Work out the finished part from the listing and answer in its coordinate system (mm). A direction names the side the tool comes from. Coordinates: 2 decimals unless noted, no trailing zeros. Write each loop counter-clockwise with the first axis right and the second up, starting at its lowest first coordinate (ties: lowest second). Pieces come first, ordered by that corner, then holes. Notation, with made-up numbers: (-1.75, 64.25) - (45.25, 64.25) arc R18 cw to (45.25, 76.25) - close; hole circle Ø4 at (43.25, 68). An arc over 180 degrees is marked (long way). Use a Markdown table: item, result. Add a question column.
(1) Given pin 1 Ø8 at (x, y) = (2.5, -25.5) entering from -Z; pin 2 Ø17 at (x, y) = (0, 0) entering from -Z; pin 3 Ø1.5 at (x, z) = (10, 2.5) entering from +Y, each flat-ended and moving along its own axis, determine where each tip first touches the part or whether it passes through.
(2) The part is cut by section D-D, the plane x = 4. Give the vertices of the cut face in (y, z) (3 decimals), then the cut area to 3 significant figures.
(3) The part is cut by section A-A, the plane z = 1.9. State how many separate pieces and enclosed holes the cut face has, then the cut area to 3 significant figures.
(4) For a pull along Y with two mould halves and no side action, classify faces 4 (the face through (-7, -35, 3.175)), 5 (the face through (0.475, -125.824, 1.61)), 6 (the face through (20.994, -97.916, 1.61)) as released by +Y, released by -Y, zero draft, split by the parting line, or undercut.
(5) A tool of negligible diameter and unlimited length cuts with its end or side. For faces 1 (the face through (-21.59, -32, 2)), 2 (the face through (-20.58, -39.69, 1.61)), 3 (the face through (-27.303, -3.698, 1.565)), from which of +Z, -Z, +X, -X, +Y, -Y can it reach the whole face along a straight path? Write none if from no direction.
(6) Find the intervals of material crossed by line 1 (Y direction, x = -10.5, z = 2.9); line 2 (Y direction, x = -9.5, z = 2.6); line 3 (Y direction, x = -16, z = 2.25), in increasing order. Write a range as from..to.
(7) The part is cut by section B-B, the plane y = -80.01. Give the vertices of the cut face in (x, z) (3 decimals).
(8) The part is cut by section C-C, the plane x = 17. Give the vertices of the cut face in (y, z) (3 decimals), then the cut area to 3 significant figures.
from build123d import *

# Parameters (mm, degrees)
SKETCH1_R            = 14.2875
SKETCH1_R_2          = 2.54
BOSS_EXTRUDE1_DEPTH  = 3.175
CUT_EXTRUDE1_DEPTH   = 162.674043733
FILLET3_R            = 6.35
BOSS_EXTRUDE3_START  = -3.175
SKETCH3_R            = 2.54
BOSS_EXTRUDE3_DEPTH  = 3.175
SKETCH6_R            = 2.54
BOSS_EXTRUDE4_DEPTH  = 3.175
FILLET2_R            = 6.35
CUT_EXTRUDE2_DEPTH   = 168.423732074
CUT_EXTRUDE3_DEPTH   = 168.423732074
CUT_EXTRUDE4_DEPTH   = 168.265702461
BOSS_EXTRUDE8_START  = -3.175
SKETCH15_R           = 2.54
BOSS_EXTRUDE8_DEPTH  = 3.175
FILLET4_R            = 2.54
BOSS_EXTRUDE9_DEPTH  = 3.175
SKETCH17_R           = 14.2875
BOSS_EXTRUDE10_DEPTH = 3.175
CUT_EXTRUDE5_DEPTH   = 131.456264953
SKETCH20_R           = 14.2875
CUT_EXTRUDE6_DEPTH   = 131.456264953
SKETCH21_R           = 2.54
CUT_EXTRUDE7_DEPTH   = 131.456264953


with BuildPart() as part:
    # Sketch1 → Boss-Extrude1 (new body)
    with BuildSketch(Plane.XY):
        with BuildLine():
            Line((-8.89, 25.4), (8.89, 25.4))
            ThreePointArc((8.89, 25.4), (17.870256121, 21.680256121), (21.59, 12.7))
            Line((21.59, 12.7), (21.59, -117.775079775))
            ThreePointArc((21.59, -117.775079775), (21.127743647, -120.388718212), (19.797058824, -122.685251408))
            Line((19.797058824, -122.685251408), (-7.952696208, -155.616779465))
            ThreePointArc((-7.952696208, -155.616779465), (-12.268297602, -157.851943494), (-16.900388255, -156.380852124))
            Line((-16.900388255, -156.380852124), (-32.439211784, -143.287061102))
            ThreePointArc((-32.439211784, -143.287061102), (-34.674375812, -138.971459708), (-33.203284443, -134.339369055))
            Line((-33.203284443, -134.339369055), (-23.382941176, -122.685251408))
            ThreePointArc((-23.382941176, -122.685251408), (-22.052256353, -120.388718212), (-21.59, -117.775079775))
            Line((-21.59, -117.775079775), (-21.59, 12.7))
            ThreePointArc((-21.59, 12.7), (-17.870256121, 21.680256121), (-8.89, 25.4))
        make_face()
        Circle(SKETCH1_R, mode=Mode.SUBTRACT)
        with Locations((0, -101.6)):
            Circle(SKETCH1_R, mode=Mode.SUBTRACT)
        with Locations((-18.532085478, -142.550133084)):
            Circle(SKETCH1_R_2, mode=Mode.SUBTRACT)
        with Locations((0, -50.8)):
            Circle(SKETCH1_R_2, mode=Mode.SUBTRACT)
    extrude(amount=BOSS_EXTRUDE1_DEPTH)

    # Sketch2 → Cut-Extrude1 (cut, through all)
    with BuildSketch(Plane.XY):
        with BuildLine():
            ThreePointArc((19.159083004, -91.647229609), (9.182340769, -50.8), (19.159083004, -9.952770391))
            ThreePointArc((19.159083004, -9.952770391), (20.973467787, -5.122670102), (21.59, 0))
            Line((21.59, 0), (27.94, 0))
            Line((27.94, 0), (27.94, -121.656687185))
            Line((27.94, -121.656687185), (-7.789552878, -164.05809836))
            Line((-7.789552878, -164.05809836), (-17.501317584, -155.874478972))
            Line((-17.501317584, -155.874478972), (16.51, -115.512152961))
            ThreePointArc((16.51, -115.512152961), (20.280273667, -109.005308906), (21.59, -101.6))
            ThreePointArc((21.59, -101.6), (20.973467787, -96.477329898), (19.159083004, -91.647229609))
        make_face()
        with BuildLine():
            Line((-21.59, -41.275), (-21.59, -60.325))
            ThreePointArc((-21.59, -60.325), (-12.065, -50.8), (-21.59, -41.275))
        make_face()
    extrude(amount=CUT_EXTRUDE1_DEPTH, mode=Mode.SUBTRACT)

    # Fillet3
    fillet3_edges = [part.edges().sort_by_distance(p)[0] for p in [
        (-21.59, -41.275, 1.5875),
        (-21.59, -60.325, 1.5875),
    ]]
    fillet(fillet3_edges, radius=FILLET3_R)

    # Sketch3 → Boss-Extrude3 (add)
    with BuildSketch(Plane.XY.offset(3.175).offset(BOSS_EXTRUDE3_START)):
        with BuildLine():
            Line((-27.351416194, -127.394768527), (-36.025496499, -137.688579))
            ThreePointArc((-36.025496499, -137.688579), (-37.217489152, -141.441859142), (-35.4063854, -144.93869507))
            Line((-35.4063854, -144.93869507), (-24.403104784, -154.210610454))
            ThreePointArc((-24.403104784, -154.210610454), (-19.771014132, -155.681701823), (-15.455412737, -153.446537795))
            Line((-15.455412737, -153.446537795), (-7.557639641, -144.073996091))
            Line((-7.557639641, -144.073996091), (-27.351416194, -127.394768527))
        make_face()
        with Locations((-18.532085478, -142.550133084)):
            Circle(SKETCH3_R, mode=Mode.SUBTRACT)
    extrude(amount=BOSS_EXTRUDE3_DEPTH)

    # Sketch6 → Boss-Extrude4 (add)
    with BuildSketch(Plane.XY.offset(3.175)):
        Polygon((-35.4063854, -144.93869507), (-63.620410749, -121.164144113), (-51.344981666, -106.596497054), (-27.065569901, -127.055545526), align=None)
        with Locations((-52.626813855, -117.972130278)):
            Circle(SKETCH6_R, mode=Mode.SUBTRACT)
    extrude(amount=-BOSS_EXTRUDE4_DEPTH)

    # Fillet2
    fillet2_edges = [part.edges().sort_by_distance(p)[0] for p in [
        (-63.620410749, -121.164144113, 1.5875),
        (-51.344981666, -106.596497054, 1.5875),
        (-27.065569901, -127.055545526, 1.5875),
    ]]
    fillet(fillet2_edges, radius=FILLET2_R)

    # Sketch7 → Cut-Extrude2 (cut, through all)
    with BuildSketch(Plane.XY.offset(3.175)):
        with BuildLine():
            Line((-21.59, 0), (-21.59, 31.75))
            Line((-21.59, 31.75), (21.59, 31.75))
            Line((21.59, 31.75), (21.59, 0))
            ThreePointArc((21.59, 0), (0, 21.59), (-21.59, 0))
        make_face()
    extrude(amount=-CUT_EXTRUDE2_DEPTH, mode=Mode.SUBTRACT)

    # Sketch10 → Cut-Extrude3 (cut, through all)
    with BuildSketch(Plane.XY.offset(3.175)):
        with BuildLine():
            Line((-18.151882461, -155.32628042), (-17.361482582, -157.512020269))
            Line((-17.361482582, -157.512020269), (-14.375706423, -156.432313955))
            Line((-14.375706423, -156.432313955), (-15.455412737, -153.446537795))
            ThreePointArc((-15.455412737, -153.446537795), (-16.679911193, -154.563907595), (-18.151882461, -155.32628042))
        make_face()
    extrude(amount=-CUT_EXTRUDE3_DEPTH, mode=Mode.SUBTRACT)

    # Sketch12 → Cut-Extrude4 (cut, through all)
    with BuildSketch(Plane.XY.offset(3.175)):
        with BuildLine():
            Line((-21.59, -101.6), (-72.39, -101.6))
            Line((-72.39, -101.6), (-72.39, -165.1))
            Line((-72.39, -165.1), (16.51, -165.1))
            Line((16.51, -165.1), (16.51, -115.512152961))
            ThreePointArc((16.51, -115.512152961), (-7.405308906, -121.880273667), (-21.59, -101.6))
        make_face()
    extrude(amount=-CUT_EXTRUDE4_DEPTH, mode=Mode.SUBTRACT)

    # Sketch15 → Boss-Extrude8 (add)
    with BuildSketch(Plane.XY.offset(3.175).offset(BOSS_EXTRUDE8_START)):
        with BuildLine():
            ThreePointArc((-34.29, -3.81), (-30.887045256, -16.51), (-21.59, -25.807045256))
            Line((-21.59, -25.807045256), (-21.59, 0))
            ThreePointArc((-21.59, 0), (-15.266435406, 15.266435406), (0, 21.59))
            Line((0, 21.59), (-8.89, 21.59))
            ThreePointArc((-8.89, 21.59), (-26.850512242, 14.150512242), (-34.29, -3.81))
        make_face()
        with Locations((-24.765, -3.81)):
            Circle(SKETCH15_R, mode=Mode.SUBTRACT)
    extrude(amount=BOSS_EXTRUDE8_DEPTH)

    # Fillet4
    fillet4_edges = [part.edges().sort_by_distance(p)[0] for p in [
        (-21.59, -25.807045256, 1.5875),
    ]]
    fillet(fillet4_edges, radius=FILLET4_R)

    # Sketch16 → Boss-Extrude9 (add, through all)
    with BuildSketch(Plane.XY.offset(3.175)):
        with BuildLine():
            Line((-21.59, -101.6), (-1.489522905, -121.700477095))
            Line((-1.489522905, -121.700477095), (4.517920132, -121.700477095))
            Line((4.517920132, -121.700477095), (21.59, -101.6))
            Line((21.59, -101.6), (21.59, -104.23906))
            ThreePointArc((21.59, -104.23906), (0, -125.82906), (-21.59, -104.23906))
            Line((-21.59, -104.23906), (-21.59, -101.6))
        make_face()
    extrude(amount=-BOSS_EXTRUDE9_DEPTH)

    # Sketch17 → Boss-Extrude10 (add, through all)
    with BuildSketch(Plane.XY.offset(3.175)):
        with Locations((0, -101.6)):
            Circle(SKETCH17_R)
    extrude(amount=-BOSS_EXTRUDE10_DEPTH)

    # Sketch19 → Cut-Extrude5 (cut, through all)
    with BuildSketch(Plane.XY.offset(3.175)):
        with BuildLine():
            Line((19.159083004, -91.647229609), (21.59, -91.647229609))
            Line((21.59, -91.647229609), (21.59, -104.23906))
            ThreePointArc((21.59, -104.23906), (20.97671132, -97.826892854), (19.159083004, -91.647229609))
        make_face()
    extrude(amount=-CUT_EXTRUDE5_DEPTH, mode=Mode.SUBTRACT)

    # Sketch20 → Cut-Extrude6 (cut, through all)
    with BuildSketch(Plane.XY.offset(3.175)):
        with Locations((0, -104.23906)):
            Circle(SKETCH20_R)
    extrude(amount=-CUT_EXTRUDE6_DEPTH, mode=Mode.SUBTRACT)

    # Sketch21 → Cut-Extrude7 (cut, through all)
    with BuildSketch(Plane.XY.offset(3.175)):
        with Locations((-9.525, -80.01)):
            Circle(SKETCH21_R)
    extrude(amount=-CUT_EXTRUDE7_DEPTH, mode=Mode.SUBTRACT)


solid = part.part
Model answer:
| question | item | result |
|---|---|---|
| 1 | pin 1 | z = 0 |
| 1 | pin 2 | through |
| 1 | pin 3 | y = 19.51 |
| 2 | outline | (-125.455, 0) - (-117.955, 0) - (-117.955, 3.175) - (-125.455, 3.175) - close; (-90.523, 0) - (-13.716, 0) - (-13.716, 3.175) - (-90.523, 3.175) - close; (13.716, 0) - (21.216, 0) - (21.216, 3.175) - (13.716, 3.175) - close |
| 2 | area | 291 mm^2 |
| 3 | separate pieces | 1 |
| 3 | enclosed holes | 5 |
| 3 | area | 4,190 mm^2 |
| 4 | face 4 | zero draft |
| 4 | face 5 | released by -Y |
| 4 | face 6 | undercut |
| 5 | face 1 | +Z, -Z, -X, -Y |
| 5 | face 2 | +Z, -Z, -X |
| 5 | face 3 | +Z, -Z |
| 6 | line 1 | -123.1..-113.93, -94.55..-82.36, -77.66..-9.69, 9.69..21.54 |
| 6 | line 2 | -123.63..-114.91, -93.57..-82.55, -77.47..-10.67, 10.67..21.58 |
| 6 | line 3 | -118.73..-58.51, -43.09..20.57 |
| 7 | outline | (-21.59, 0) - (-12.065, 0) - (-12.065, 3.175) - (-21.59, 3.175) - close; (-6.985, 0) - (14.135, 0) - (14.135, 3.175) - (-6.985, 3.175) - close |
| 8 | outline | (-117.548, 0) - (-87.191, 0) - (-87.191, 3.175) - (-117.548, 3.175) - close; (-14.409, 0) - (13.309, 0) - (13.309, 3.175) - (-14.409, 3.175) - close |
| 8 | area | 184 mm^2 |
